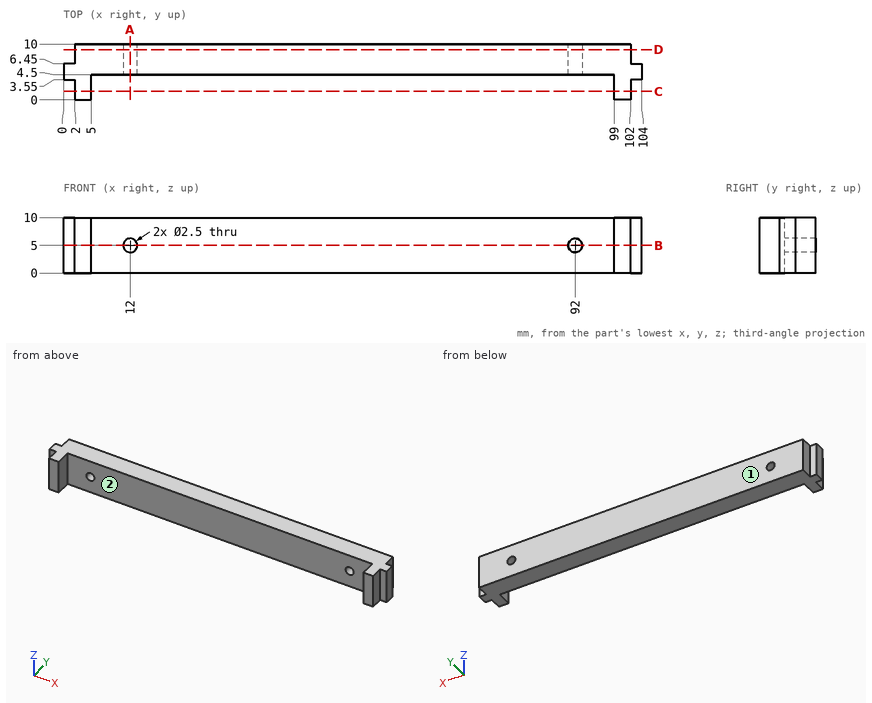
The drawing under review shows one solid part. Ordinate dimensions are in mm from its lowest x, y, z. Coordinates: 2 decimals unless noted, no trailing zeros. Order: outer loops, then holes, each group sorted by start corner. A loop starts at its lowest first (then second) coordinate and runs counter-clockwise, first axis right, second up. Notation, with made-up numbers: M 43,55 L 53,55 A34 cw 53,88 Z; hole C 3.25,22.5 d8. An arc over 180 degrees is marked long. One line per question, with ' | ' between items.
(1) The part is to be moulded in two halves that separate along X. For the marked faces 1 and 2, say which applies: +X half, -X half, draft (parallel to the pull), parting line (faces both ways), or undercut.
Geometry results:
face 1: draft | face 2: undercut
(2) For probe 1 along Z at (x, y) = (12, 8.05); probe 2 along X at (y, z) = (4.25, 2.5); probe 3 along X at (y, z) = (3, 7.75), list the stretches that pass through material, from the lowest coordinate up. Write a range as from..to.
Geometry results:
probe 1: z = 0..3.75, 6.25..10 | probe 2: x = 0..5, 99..104 | probe 3: x = 2..5, 99..102
(3) Add section B-B, the plane z = 5. Write out the cut boundary in (x, y), then the cut area to 3 significant figures.
Geometry results:
outline: M 0,3.55 L 2,3.55 L 2,0 L 5,0 L 5,4.5 L 10.75,4.5 L 10.75,10 L 2,10 L 2,6.45 L 0,6.45 Z; M 13.25,4.5 L 90.75,4.5 L 90.75,10 L 13.25,10 Z; M 93.25,4.5 L 99,4.5 L 99,0 L 102,0 L 102,3.55 L 104,3.55 L 104,6.45 L 102,6.45 L 102,10 L 93.25,10 Z | area: 561 mm²
(4) Add section C-C, the plane y = 1.5. Write out the cut boundary in (x, z), then the cut area to 3 significant figures.
Geometry results:
outline: M 2,0 L 5,0 L 5,10 L 2,10 Z; M 99,0 L 102,0 L 102,10 L 99,10 Z | area: 60.0 mm²
(5) Add section A-A, the plane x = 12. Write out the cut boundary in (y, z), then the cut area to 4 significant figures.
Geometry results:
outline: M 4.5,0 L 10,0 L 10,3.75 L 4.5,3.75 Z; M 4.5,6.25 L 10,6.25 L 10,10 L 4.5,10 Z | area: 41.25 mm²
(6) Add section D-D, the plane y = 9. Write out the cut boundary in (x, z), then the cut area to 3 significant figures.
Geometry results:
outline: M 2,0 L 102,0 L 102,10 L 2,10 Z; hole C 12,5 d2.5; hole C 92,5 d2.5 | area: 990 mm²
(7) Insertion check: pin 1 (1.1 mm diameter, centred on y = 1, z = 7, fed in from -X); pin 2 (1 mm diameter, centred on x = 103, z = 2.5, fed in from +Y); pin 3 (1 mm diameter, centred on x = 82, y = 7, fed in from -Z); pin 4 (1.6 mm diameter, centred on x = 103.5, z = 4, fed in from -Y). Each pin has a flat end and moves straight along its axis. Give the tip position at first contact, or say it passes through.
Geometry results:
pin 1: stops at x = 2 | pin 2: stops at y = 6.45 | pin 3: stops at z = 0 | pin 4: stops at y = 3.55
